Part print with two shaded views. Sizes in mm from the minimum x, y, z corner. A direction names the side the tool comes from. Round coordinates to 2 decimals unless told otherwise and drop trailing zeros. Order: outer loops, then holes, each group sorted by start corner. A loop starts at its lowest first (then second) coordinate and runs counter-clockwise, first axis right, second up. Notation, with made-up numbers: M 84,3 L 140,3 A3 ccw 140,8 Z; hole C -6.5,2.25 d9. An arc over 180 degrees is marked long. Answer as a JSON object with one key per item and string values.
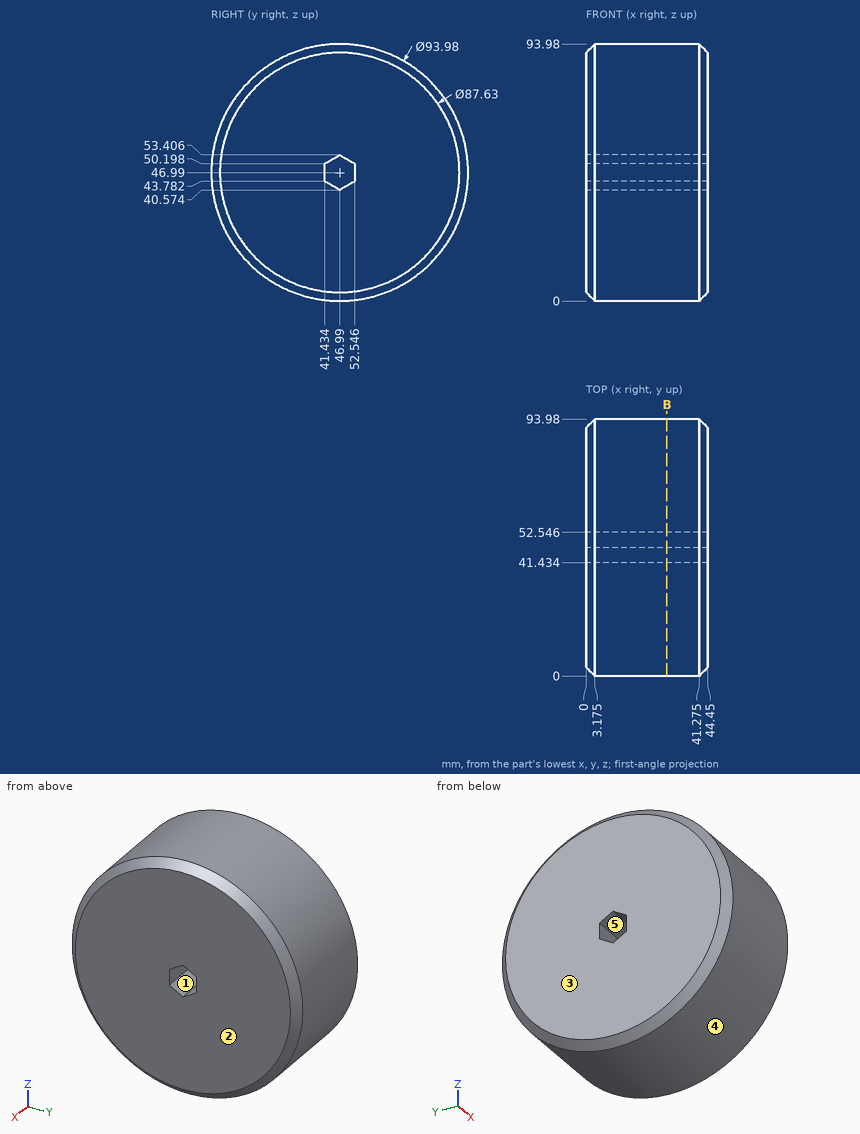
Item 1: Wall check: line 1 along Y through (x, z) = (35.5, 51) (1 decimal); line 2 along Y through (x, z) = (19, 42.5) (1 decimal); line 3 along Z through (x, y) = (36, 48.5) (1 decimal). Give the ranges that are in metal, low to high. Write a range as [from, to].
Worked answers:
{"line 1": "y = [0.2, 42.8], [51.2, 93.8]", "line 2": "y = [0.2, 43.7], [50.3, 93.8]", "line 3": "z = [0, 41.4], [52.5, 94]"}
Item 2: Two-plate mould, pull along Z, no slides. Class the marked faces 3, 4 and 5: released by +Z, released by -Z, zero draft, split by the parting line, or undercut.
Worked answers:
{"face 3": "zero draft", "face 4": "split by the parting line", "face 5": "undercut"}
Item 3: Saw through at B-B on x = 29.5. List the corners of the cut face in (y, z), and give its area (3 significant figures).
Worked answers:
{"outline": "C 46.99,46.99 d93.98; hole M 41.43,43.78 L 46.99,40.57 L 52.55,43.78 L 52.55,50.2 L 46.99,53.41 L 41.43,50.2 Z", "area": "6,830 mm2"}
Item 4: Drop flat-ended pins along their axis: pin 1 Ø4 at (x, z) = (37, 30.5) entering from -Y; pin 2 Ø3 at (x, y) = (32, 57.5) entering from +Z; pin 3 Ø1 at (x, y) = (27.5, 36.5) entering from +Z. Give the stop position or say it passes through.
Worked answers:
{"pin 1": "stops at y = 2.29", "pin 2": "stops at z = 93.11", "pin 3": "stops at z = 92.91"}
Item 5: 3-axis set-ups, long thin cutter, end or side, ignore diameter. For the marked faces 1 and 2: which of +Z, -Z, +X, -X, +Y, -Y reach the whole face in a straight line?
Worked answers:
{"face 1": "+X, -X", "face 2": "+Z, -Z, +X, +Y, -Y"}
